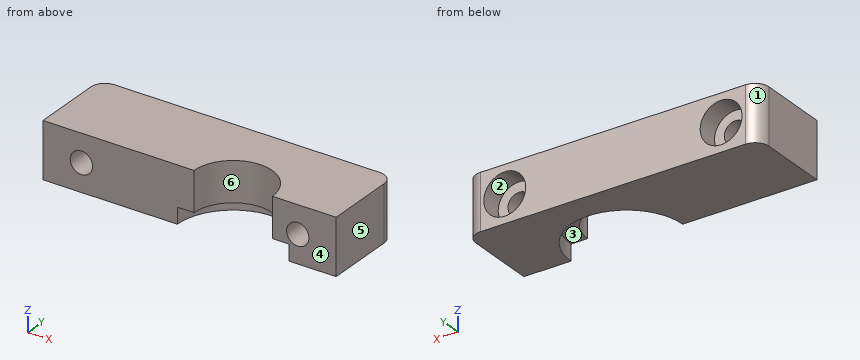
from build123d import *

# Parameters (mm, degrees)
SKETCH007_R  = 1.6
PAD007_DEPTH = 12
SKETCH005_R  = 8
PAD005_DEPTH = 2.3
SKETCH008_R  = 3
PAD008_DEPTH = 3
PAD_DEPTH    = 8
FILLET_R     = 2


with BuildPart() as hotendmount02:
    # Sketch007 → Pad007 (new body)
    with BuildSketch(Plane.XZ):
        with Locations((5.5, 4)):
            Circle(SKETCH007_R)
        with Locations((36.5, 4)):
            Circle(SKETCH007_R)
    extrude(amount=-PAD007_DEPTH)


with BuildPart() as hotendmount:
    # Sketch005 → Pad005 (new body)
    with BuildSketch(Plane.XY):
        with Locations((27.25, 0)):
            Circle(SKETCH005_R)
    extrude(amount=PAD005_DEPTH)


with BuildPart() as cutblock:
    # Sketch008 → Pad008 (new body)
    with BuildSketch(Plane.XZ.offset(-9)):
        with Locations((5.5, 4)):
            Circle(SKETCH008_R)
        with Locations((36.5, 4)):
            Circle(SKETCH008_R)
    extrude(amount=-PAD008_DEPTH)

    # Fusion: union HotEndMount02, HotEndMount
    add(hotendmount02.part)
    add(hotendmount.part)


with BuildPart() as fillet_body:
    # Sketch → Pad (new body)
    with BuildSketch(Plane.XY):
        with BuildLine():
            Line((0, 12), (42, 12))
            Line((42, 12), (42, 0))
            Line((32.85, 0), (42, 0))
            ThreePointArc((32.85, 0), (27.25, 5.6), (21.65, 0))
            Line((21.65, 0), (0, 0))
            Line((0, 0), (0, 12))
        make_face()
    extrude(amount=PAD_DEPTH)

    # Cut: cut CutBlock
    add(cutblock.part, mode=Mode.SUBTRACT)

    # Fillet
    fillet_edges = [fillet_body.edges().sort_by_distance(p)[0] for p in [
        (42, 12, 4),
        (0, 12, 4),
    ]]
    fillet(fillet_edges, radius=FILLET_R)


solid = fillet_body.part
Verification items for the finished model (mm, model axes). Face numbers are marked on the shaded views. A direction names the side the tool comes from. Round coordinates to 2 decimals unless told otherwise and drop trailing zeros. Write each loop counter-clockwise with the first axis right and the second up, starting at its lowest first coordinate (ties: lowest second). Pieces come first, ordered by that corner, then holes.
(1) Section check B-B (z = 4). Enter the section's corners in (x, y), plus the area to 3 significant figures.
Returned:
outline: (0, 0) - (3.9, 0) - (3.9, 9) - (2.5, 9) - (2.5, 12) - (2, 12) arc R2 ccw to (0, 10) - close; (7.1, 0) - (21.65, 0) arc R5.6 cw to (32.85, 0) - (34.9, 0) - (34.9, 9) - (33.5, 9) - (33.5, 12) - (8.5, 12) - (8.5, 9) - (7.1, 9) - close; (38.1, 0) - (42, 0) - (42, 10) arc R2 ccw to (40, 12) - (39.5, 12) - (39.5, 9) - (38.1, 9) - close
area: 359 mm2
(2) Section check A-A (x = 5.5). Enter the section's corners in (y, z).
Returned:
outline: (0, 0) - (12, 0) - (12, 1) - (9, 1) - (9, 2.4) - (0, 2.4) - close; (0, 5.6) - (9, 5.6) - (9, 7) - (12, 7) - (12, 8) - (0, 8) - close
(3) Section check C-C (y = 2.75). Enter the section's corners in (x, z).
Returned:
outline: (0, 0) - (19.74, 0) - (19.74, 2.3) - (22.37, 2.3) - (22.37, 8) - (0, 8) - close; (32.13, 2.3) - (34.76, 2.3) - (34.76, 0) - (42, 0) - (42, 8) - (32.13, 8) - close; hole circle Ø3.2 at (5.5, 4); hole circle Ø3.2 at (36.5, 4)
(4) Access from +Z, -Z, +X, -X, +Y, -Y to the whole of each face (thin tool, end or side, straight path). Record for the marked faces 1, 2 and 3.
Returned:
face 1: +Z, -Z, -X, +Y
face 2: +Y
face 3: -Z, -Y
(5) Material ranges on line 1 (Z direction, x = 36.5, y = 11.3); line 2 (Z direction, x = 5.5, y = 5.75); line 3 (X direction, y = 9.25, z = 2.25), recorded low to high.
Returned:
line 1: z = 0 to 1, 7 to 8
line 2: z = 0 to 2.4, 5.6 to 8
line 3: x = 0 to 3.06, 7.94 to 34.06, 38.94 to 42
(6) Section check D-D (z = 0.5). Enter the section's corners in (x, y).
Returned:
outline: (0, 0) - (19.25, 0) arc R8 cw to (35.25, 0) - (42, 0) - (42, 10) arc R2 ccw to (40, 12) - (2, 12) arc R2 ccw to (0, 10) - close
(7) Mould release check, pull along X, two halves, no side actions. Record for the marked faces 4, 5 and 6: pulls with the +X half, pulls with the -X half, needs draft (parallel to the pull), parting line crosses it, or undercut.
Returned:
face 4: needs draft
face 5: pulls with the +X half
face 6: undercut
